Input: part model. Units: mm. Frame: model coordinates. Coordinates: 2 decimals unless noted, no trailing zeros. Write each loop counter-clockwise with the first axis right and the second up, starting at its lowest first coordinate (ties: lowest second). Pieces come first, ordered by that corner, then holes. Notation, with made-up numbers: (36.5, -1) -> (77.5, -1) arc R14 cw to (77.5, 4) -> close; hole circle Ø5 at (64, -23.5). An arc over 180 degrees is marked (long way). Use one line per item in the form item = value. Start each with the question number.
(1) Cut plane D-D on z = 14. Return the cut outline in (x, y).
(2) Ray query, line 1 along Z through (x, y) = (2, -33.5); line 2 along X through (y, z) = (-5.5, -9); line 3 along Z through (x, y) = (4.5, -39.5). Return the intervals inside material, ascending.
(3) Cut plane B-B on z = 0.5. Return the cut outline in (x, y).
(4) Cut plane C-C on z = -7. Return the cut outline in (x, y), plus the area to 3 significant figures.
(5) Pull-direction query (Z, two-part tool) for faces 1 (the face through (-1, 0, 0)), 2 (the face through (5.453, -39.847, 0.077)), 3 (the face through (1, -21, -17.5)); classes: released by +Z, released by -Z, zero draft, split by the parting line, or undercut.
(6) First-contact query: pin 1 (8 mm diameter, centred on y = -33, z = -0.5, fed in from -X); pin 2 (3 mm diameter, centred on x = 8, y = -35, fed in from -Z); pin 3 (1 mm diameter, centred on y = -25, z = 11, fed in from +X). Flat tips, straight axial feed; report the tip coordinate or a pass-through.
(7) Cut plane A-A on y = -25. Return the cut outline in (x, z), plus the area to 3 significant figures.
```python
from build123d import *

# Parameters (mm, degrees)
EXTRUSION1_DEPTH        = 17.5
CONG_1_R                = 4
ENL_V_MAT_EXTRU_1_DEPTH = 35


with BuildPart() as part:
    # Esquisse1 → Extrusion1 (new body, symmetric)
    with BuildSketch(Plane.XY):
        with BuildLine():
            Line((0, 0), (-3.006199407, 0))
            ThreePointArc((-3.006199407, 0), (-1.239978733, -23.393785135), (6.853974171, -45.413699867))
            Line((6.853974171, -45.413699867), (9.5, -44))
            ThreePointArc((9.5, -44), (1.671662982, -22.664640947), (0, 0))
        make_face()
    extrude(amount=EXTRUSION1_DEPTH, both=True)

    # Congé1
    cong_1_edges = [part.edges().sort_by_distance(p)[0] for p in [
        (-1.503099703, 0, 17.5),
        (-1.503099703, 0, -17.5),
        (8.176987086, -44.706849934, -17.5),
        (8.176987086, -44.706849934, 17.5),
    ]]
    fillet(cong_1_edges, radius=CONG_1_R)

    # Esquisse2 → Enlèv. mat.-Extru.1 (cut)
    with BuildSketch(Plane(origin=(0, 0, 0), x_dir=(0, 0, 1), z_dir=(-0.977476134, -0.211045984, 0))):
        with BuildLine():
            Line((-3.5, -36.601432597), (-3.5, -8.601432597))
            ThreePointArc((-3.5, -8.601432597), (0, -5.101432597), (3.5, -8.601432597))
            Line((3.5, -8.601432597), (3.5, -36.601432597))
            ThreePointArc((3.5, -36.601432597), (0, -40.101432597), (-3.5, -36.601432597))
        make_face()
    extrude(amount=ENL_V_MAT_EXTRU_1_DEPTH, mode=Mode.SUBTRACT)


solid = part.part
```
Values:
q1.outline = (-3.01, -0.03) arc R85 ccw to (6.84, -45.39) -> (9.49, -43.97) arc R82 cw to (0, -0.03) -> close
q2.line_1 = -17.5 to -3.5, 3.5 to 17.5
q2.line_2 = -3.18 to -0.18
q2.line_3 = -17.5 to -1.87, 1.87 to 17.5
q3.outline = (-3.17, -5.94) -> (-0.18, -5.29) arc R82 cw to (0, 0) -> (-3.01, 0) arc R85 ccw to start; (4.24, -40.07) arc R85 ccw to (6.85, -45.41) -> (9.5, -44) arc R82 cw to (7.24, -39.43) -> close
q4.outline = (-3.01, 0) arc R85 ccw to (6.85, -45.41) -> (9.5, -44) arc R82 cw to (0, 0) -> close
q4.area = 139 mm2
q5.face_1 = zero draft
q5.face_2 = undercut
q5.face_3 = released by -Z
q6.pin_1 = 0.58
q6.pin_2 = through
q6.pin_3 = 2.34
q7.outline = (-0.87, -17.5) -> (2.21, -17.5) -> (2.21, -3.5) -> (-0.87, -3.5) -> close; (-0.87, 3.5) -> (2.21, 3.5) -> (2.21, 17.5) -> (-0.87, 17.5) -> close
q7.area = 86.4 mm2
